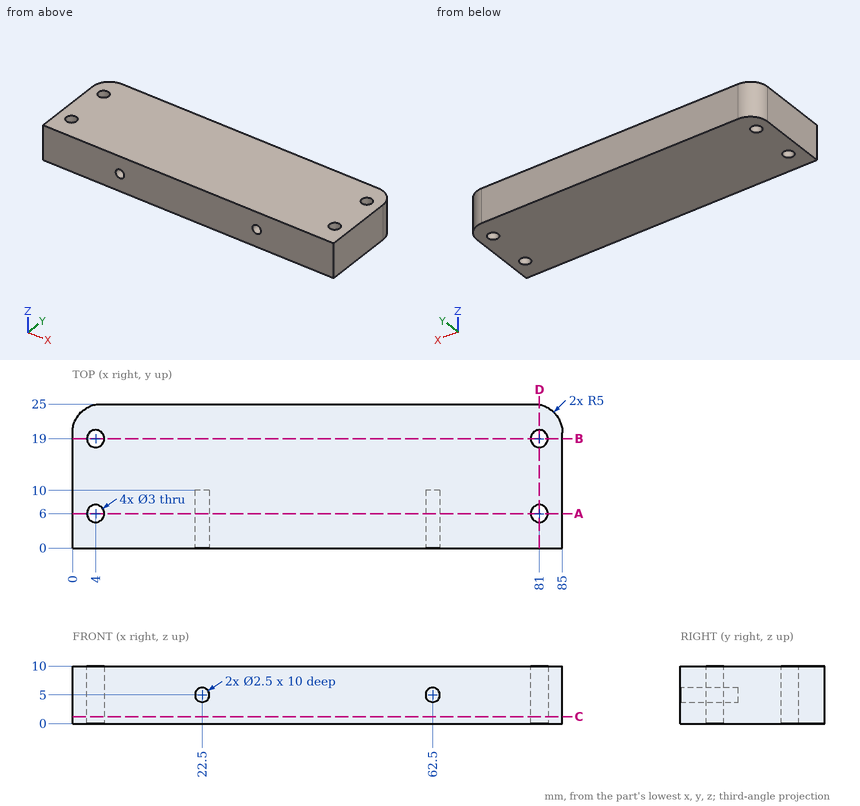
Job drawing, mm, ordinate dimensions from the low corner. One solid piece. Coordinates: 2 decimals unless noted, no trailing zeros. Write each loop counter-clockwise with the first axis right and the second up, starting at its lowest first coordinate (ties: lowest second). Pieces come first, ordered by that corner, then holes. Notation, with made-up numbers: M -5,23 L 38,23 A17 ccw 38,54 Z; hole C 52.5,66 d4. An arc over 180 degrees is marked long. Answer as a JSON object with one key per item and string values. Group by question number.
1) Pin check, flat tips, straight feed: pin 1 Ø3 at (x, z) = (22.5, 5) entering from -Y; pin 2 Ø1.8 at (x, y) = (81, 6) entering from +Z; pin 3 Ø1.2 at (x, z) = (22.5, 4.5) entering from -Y. Stop position of each tip, or through.
2) Saw through at D-D (x = 81). Write the cut outline in (y, z).
3) Saw through at C-C (z = 1.25). Write the cut outline in (x, y), plus the area to 3 significant figures.
4) Saw through at B-B (y = 19). Write the cut outline in (x, z).
5) Saw through at A-A (y = 6). Write the cut outline in (x, z).
6) Wall check: line 1 (Y direction, x = 80, z = 3.75); line 2 (Y direction, x = 4, z = 6); line 3 (X direction, y = 6.5, z = 5). Give the ranges that are in metal, low to high. Write a range as from..to.
Values follow:
{
 "1": {"pin 1": "stops at y = 0", "pin 2": "passes through", "pin 3": "stops at y = 10"},
 "2": {"outline": "M 0,0 L 4.5,0 L 4.5,10 L 0,10 Z; M 7.5,0 L 17.5,0 L 17.5,10 L 7.5,10 Z; M 20.5,0 L 24.9,0 L 24.9,10 L 20.5,10 Z"},
 "3": {"outline": "M 0,0 L 85,0 L 85,20 A5 ccw 80,25 L 5,25 A5 ccw 0,20 Z; hole C 4,6 d3; hole C 4,19 d3; hole C 81,6 d3; hole C 81,19 d3", "area": "2,090 mm2"},
 "4": {"outline": "M 0,0 L 2.5,0 L 2.5,10 L 0,10 Z; M 5.5,0 L 79.5,0 L 79.5,10 L 5.5,10 Z; M 82.5,0 L 85,0 L 85,10 L 82.5,10 Z"},
 "5": {"outline": "M 0,0 L 2.5,0 L 2.5,10 L 0,10 Z; M 5.5,0 L 79.5,0 L 79.5,10 L 5.5,10 Z; M 82.5,0 L 85,0 L 85,10 L 82.5,10 Z; hole C 22.5,5 d2.5; hole C 62.5,5 d2.5"},
 "6": {"line 1": "y = 0..4.88, 7.12..17.88, 20.12..25", "line 2": "y = 0..4.5, 7.5..17.5, 20.5..24.9", "line 3": "x = 0..2.59, 5.41..21.25, 23.75..61.25, 63.75..79.59, 82.41..85"}
}
